Input: part model. Units: mm. Frame: model coordinates. A direction names the side the tool comes from. Give positions to 0.01 mm unless a question says otherwise; leave off trailing zeros. Write each loop counter-clockwise with the first axis right and the second up, starting at its lowest first coordinate (ties: lowest second). Pieces come first, ordered by that corner, then holes.
```python
from build123d import *

# Parameters (mm, degrees)
BOSS_EXTRUDE1_DEPTH = 3


with BuildPart() as part:
    # Sketch1 → Boss-Extrude1 (new body)
    with BuildSketch(Plane.XY):
        Polygon((471.00000486, 293.272073149), (467.272082799, 296.99999521), (438.727926921, 296.99999521), (435.00000486, 293.272073149), (435.00000486, 264.727917272), (438.727926921, 260.99999521), (467.272082799, 260.99999521), (471.00000486, 264.727917272), align=None)
        Polygon((454.50000486, 274.49999521), (454.50000486, 277.49999521), (457.50000486, 277.49999521), (457.50000486, 280.49999521), (454.50000486, 280.49999521), (454.50000486, 283.49999521), (451.50000486, 283.49999521), (451.50000486, 280.49999521), (448.50000486, 280.49999521), (448.50000486, 277.49999521), (451.50000486, 277.49999521), (451.50000486, 274.49999521), align=None, mode=Mode.SUBTRACT)
    extrude(amount=BOSS_EXTRUDE1_DEPTH)


solid = part.part
```
Item 1: Section B-B (z = 2.3). Return loops of the section in (x, y).
Item 2: Set-up query: faces 4 (the flat face through (471, 279, 1)), 5 (the flat face through (457.5, 279, 1)). Return all of +Z, -Z, +X, -X, +Y, -Y with unobstructed straight access to the full face (end or side cutting, diameter ignored); none if empty.
Item 3: Pin query (flat end, axial travel): pin 1 (3 mm diameter, centred on x = 465.5, y = 292.5, fed in from -Z). Return the tip coordinate at first contact, or that it passes through.
Item 4: Ray query, line 1 (Y direction, x = 453.5, z = 0.2); line 2 (Y direction, x = 449.5, z = 1.2); line 3 (X direction, y = 278.5, z = 0.75). Return the intervals inside material, ascending.
Item 5: Section A-A (x = 449). Return loops of the section in (y, z).
Item 6: Mould query, pull axis X, two halves, no side actions, for faces 1 (the flat face through (436.84, 262.89, 1.48)), 2 (the flat face through (457, 275, 3)), 3 (the flat face through (451.5, 282, 1)). Classes: +X half, -X half, draft (parallel to the pull), parting line (faces both ways), or undercut.
Item 7: Section C-C (y = 283). Return loops of the section in (x, z).
Solved:
1. outline: (435, 264.73) - (438.73, 261) - (467.27, 261) - (471, 264.73) - (471, 293.27) - (467.27, 297) - (438.73, 297) - (435, 293.27) - close; hole (448.5, 277.5) - (451.5, 277.5) - (451.5, 274.5) - (454.5, 274.5) - (454.5, 277.5) - (457.5, 277.5) - (457.5, 280.5) - (454.5, 280.5) - (454.5, 283.5) - (451.5, 283.5) - (451.5, 280.5) - (448.5, 280.5) - close
2. face 4: +Z, -Z, +X, +Y, -Y
2. face 5: +Z, -Z
3. pin 1: stops at z = 0
4. line 1: y = 261 to 274.5, 283.5 to 297
4. line 2: y = 261 to 277.5, 280.5 to 297
4. line 3: x = 435 to 448.5, 457.5 to 471
5. outline: (261, 0) - (277.5, 0) - (277.5, 3) - (261, 3) - close; (280.5, 0) - (297, 0) - (297, 3) - (280.5, 3) - close
6. face 1: -X half
6. face 2: draft
6. face 3: undercut
7. outline: (435, 0) - (451.5, 0) - (451.5, 3) - (435, 3) - close; (454.5, 0) - (471, 0) - (471, 3) - (454.5, 3) - close
